Part model, mm, in its own coordinate system. A direction names the side the tool comes from. Round coordinates to 2 decimals unless told otherwise and drop trailing zeros. Loops run counter-clockwise (first coordinate to the right, second up) from the corner with the lowest first, then second, coordinate; pieces in that order, holes last. Notation, with made-up numbers: (-39, 84.5) -> (-16, 84.5) arc R12 cw to (-16, 106.5) -> close; hole circle Ø7 at (-29, 79.5). An arc over 180 degrees is marked (long way). Answer as a JSON object with one key per item and string values. Group by question number.
from build123d import *

# Parameters (mm, degrees)
F0_W      = 160
F0_H      = 38
F1_DEPTH  = 1
F2_W      = 160
F2_H      = 32
F3_DEPTH  = 1
F4_W      = 160
F4_H      = 32
F5_DEPTH  = 1
F7_DEPTH  = 40.001
F8_DEPTH  = 40.001
F9_W      = 128
F9_H      = 1
F10_DEPTH = 38


with BuildPart() as f1:
    # F0 (on Top) → F1 (new body)
    with BuildSketch(Plane.XY):
        Rectangle(F0_W, F0_H)
    extrude(amount=F1_DEPTH)

    # F2 (on face) → F3 (join)
    with BuildSketch(Plane.XZ.offset(19)):
        with Locations((0, 16)):
            Rectangle(F2_W, F2_H)
    extrude(amount=F3_DEPTH)

    # F4 (on face) → F5 (join)
    with BuildSketch(Plane(origin=(0, 19, 0), x_dir=(-1, 0, 0), z_dir=(0, 1, 0))):
        with Locations((0, 16)):
            Rectangle(F4_W, F4_H)
    extrude(amount=F5_DEPTH)

    # F6 (on face) → F7 (cut, through all)
    with BuildSketch(Plane.XZ.offset(20)):
        with BuildLine():
            ThreePointArc((-80, 16), (-75.313708, 27.313708), (-64, 32))
            Line((-64, 32), (-80, 32))
            Line((-80, 32), (-80, 16))
        make_face()
    extrude(amount=-F7_DEPTH, mode=Mode.SUBTRACT)

    # F6 (on face) → F8 (cut, through all)
    with BuildSketch(Plane.XZ.offset(20)):
        with BuildLine():
            Line((80, 32), (64, 32))
            ThreePointArc((64, 32), (75.313708, 27.313708), (80, 16))
            Line((80, 16), (80, 32))
        make_face()
    extrude(amount=-F8_DEPTH, mode=Mode.SUBTRACT)

    # F9 (on face) → F10 (join)
    with BuildSketch(Plane(origin=(0, -19, 0), x_dir=(-1, 0, 0), z_dir=(0, 1, 0))):
        with Locations((0, 31.5)):
            Rectangle(F9_W, F9_H)
    extrude(amount=F10_DEPTH)


solid = f1.part
Item 1: Two-plate mould, pull along Z, no slides. Class faces 3 (the face through (-1, -19, 17)), 4 (the face through (-75.437, 19.493, 27.189)), 5 (the face through (1, 20, 16)): pulls with the +Z half, pulls with the -Z half, needs draft (parallel to the pull), parting line crosses it, or undercut.
Item 2: Which spindle directions (+Z, -Z, +X, -X, +Y, -Y) get a long thin tool onto all of the face, cutting with end or side? Do faces 1 (the face through (-1, 0, 1)), 2 (the face through (1, 0, 32)). Say none if no direction does.
Item 3: Band-saw the part on B-B, the plane x = 19. List the corners of the cut face in (y, z), plus the area to 3 significant figures.
Item 4: Band-saw the part on C-C, the plane y = -14. List the corners of the cut face in (x, z).
Item 5: Drill centre lines: line 1 (Y direction, x = 27, z = 23); line 2 (Z direction, x = 34, y = -0.5); line 3 (Z direction, x = 71, y = 10). Where is each one in solid material? Low to high.
Item 6: Drop flat-ended pins along their axis: pin 1 Ø10 at (x, y) = (-2, 13) entering from -Z; pin 2 Ø0.5 at (y, z) = (7.5, 31.5) entering from +X; pin 3 Ø1.1 at (y, z) = (3.5, 31.5) entering from -X. Give the stop position or say it passes through.
Item 7: Band-saw the part on D-D, the plane x = -66. List the corners of the cut face in (y, z).
Item 8: Band-saw the part on A-A, the plane z = 3. List the corners of the cut face in (x, y), plus the area to 3 significant figures.
Entries:
{
 "1": {"face 3": "undercut", "face 4": "pulls with the +Z half", "face 5": "needs draft"},
 "2": {"face 1": "+X, -X", "face 2": "+Z, +X, -X, +Y, -Y"},
 "3": {"outline": "(-20, 0) -> (20, 0) -> (20, 32) -> (-20, 32) -> close; hole (-19, 1) -> (19, 1) -> (19, 31) -> (-19, 31) -> close", "area": "140 mm²"},
 "4": {"outline": "(-80, 0) -> (80, 0) -> (80, 1) -> (-80, 1) -> close; (-64, 31) -> (64, 31) -> (64, 32) -> (-64, 32) -> close"},
 "5": {"line 1": "-20 to -19, 19 to 20", "line 2": "0 to 1, 31 to 32", "line 3": "0 to 1"},
 "6": {"pin 1": "z = 0", "pin 2": "x = 64", "pin 3": "x = -64"},
 "7": {"outline": "(-20, 0) -> (20, 0) -> (20, 31.87) -> (19, 31.87) -> (19, 1) -> (-19, 1) -> (-19, 31.87) -> (-20, 31.87) -> close"},
 "8": {"outline": "(-80, -20) -> (80, -20) -> (80, -19) -> (-80, -19) -> close; (-80, 19) -> (80, 19) -> (80, 20) -> (-80, 20) -> close", "area": "320 mm²"}
}
